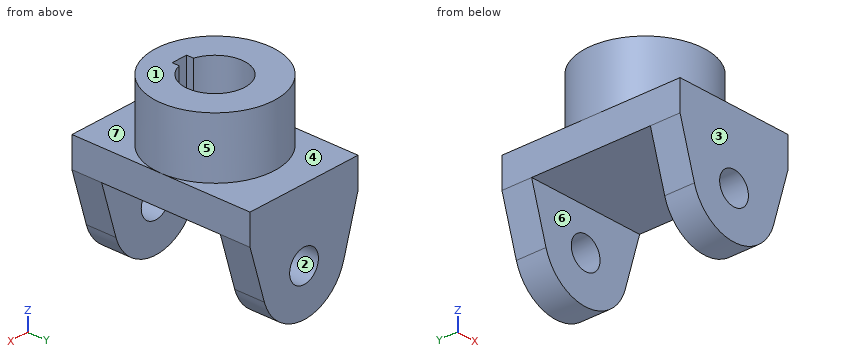
```python
from build123d import *

# Parameters (mm, degrees)
SKETCH1_W           = 60
SKETCH1_H           = 90
BOSS_EXTRUDE1_DEPTH = 7.5
SKETCH2_R           = 30
BOSS_EXTRUDE4_DEPTH = 30
SKETCH3_R           = 8
BOSS_EXTRUDE5_DEPTH = 15


with BuildPart() as part:
    # Sketch1 → Boss-Extrude1 (new body, symmetric)
    with BuildSketch(Plane.XY):
        Rectangle(SKETCH1_W, SKETCH1_H)
    extrude(amount=BOSS_EXTRUDE1_DEPTH, both=True)

    # Sketch2 → Boss-Extrude4 (add)
    with BuildSketch(Plane.XY.offset(7.5)):
        Circle(SKETCH2_R)
        with BuildLine():
            Line((4, -18), (0, -18))
            Line((0, -18), (-4, -18))
            Line((-4, -18), (-4, -15))
            Line((-4, -15), (-4, -14.456832295))
            ThreePointArc((-4, -14.456832295), (-9.082951062, 11.937336386), (15, 0))
            ThreePointArc((15, 0), (11.937336386, -9.082951062), (4, -14.456832295))
            Line((4, -14.456832295), (4, -18))
        make_face(mode=Mode.SUBTRACT)
    extrude(amount=BOSS_EXTRUDE4_DEPTH)

    # Sketch3 → Boss-Extrude5 (add)
    with BuildSketch(Plane(origin=(0, 45, 0), x_dir=(1, 0, 0), z_dir=(0, 1, 0))):
        with BuildLine():
            Line((-22.03289839, 34.099347585), (-30, 7.5))
            Line((-30, 7.5), (-11.357816691, 7.5))
            ThreePointArc((-11.357816691, 7.5), (-21.345170095, 18.933570545), (-22.03289839, 34.099347585))
        make_face()
        with BuildLine():
            Line((30, 7.5), (22.03289839, 34.099347585))
            ThreePointArc((22.03289839, 34.099347585), (22.756940293, 30.834916568), (23, 27.5))
            ThreePointArc((23, 27.5), (19.877497125, 15.929126738), (11.357816692, 7.5))
            Line((11.357816692, 7.5), (30, 7.5))
        make_face()
        with BuildLine():
            ThreePointArc((22.03289839, 34.099347585), (0, 50.5), (-22.03289839, 34.099347585))
            ThreePointArc((-22.03289839, 34.099347585), (-21.345170095, 18.933570545), (-11.357816691, 7.5))
            Line((-11.357816691, 7.5), (11.357816692, 7.5))
            ThreePointArc((11.357816692, 7.5), (19.877497125, 15.929126738), (23, 27.5))
            ThreePointArc((23, 27.5), (22.756940293, 30.834916568), (22.03289839, 34.099347585))
        make_face()
        with Locations((0, 27.5)):
            Circle(SKETCH3_R, mode=Mode.SUBTRACT)
    boss_extrude5 = extrude(amount=-BOSS_EXTRUDE5_DEPTH)

    # Mirror1: Boss-Extrude5 across plane
    add(boss_extrude5.mirror(Plane.ZX))


solid = part.part
```
Input: part model. Units: mm. Frame: model coordinates. Face numbers are marked on the shaded views. A direction names the side the tool comes from. Coordinates: 2 decimals unless noted, no trailing zeros. Loops run counter-clockwise (first coordinate to the right, second up) from the corner with the lowest first, then second, coordinate; pieces in that order, holes last. Notation, with made-up numbers: M 76,5 L 135,5 A12 ccw 135,16 Z; hole C -10,33.25 d3. An arc over 180 degrees is marked long. Answer in a Markdown table with one row per item.
1. Reachability of the marked faces 4, 5, 6 and 7 from +Z, -Z, +X, -X, +Y, -Y: full face, straight path, thin tool, end or side. Return the list, or none.
Response:
| item | result |
|---|---|
| face 4 | +Z, +Y |
| face 5 | +Z |
| face 6 | -Z, +X, -X |
| face 7 | +Z, -Y |
2. First-contact query: pin 1 (2 mm diameter, centred on x = 18.5, z = 14.5, fed in from +Y); pin 2 (2 mm diameter, centred on x = -12, z = 19.5, fed in from +Y); pin 3 (5 mm diameter, centred on x = -22.5, y = 14, fed in from -Z). Flat tips, straight axial feed; report the tip coordinate or a pass-through.
Response:
| item | result |
|---|---|
| pin 1 | stops at y = 24.37 |
| pin 2 | stops at y = 27.91 |
| pin 3 | stops at z = -7.5 |
3. Section C-C, the plane y = 18. Output: boundary loops of the cut face in (x, z), then the cut area to 3 significant figures.
Response:
| item | result |
|---|---|
| outline | M -30,-7.5 L 30,-7.5 L 30,7.5 L 24,7.5 L 24,37.5 L -24,37.5 L -24,7.5 L -30,7.5 Z |
| area | 2,340 mm2 |
4. Section D-D, the plane z = -27.5. Output: boundary loops of the cut face in (x, y), then the cut area to 3 significant figures.
Response:
| item | result |
|---|---|
| outline | M -24.01,-45 L -8,-45 L -8,-30 L -24.01,-30 Z; M -24.01,30 L -8,30 L -8,45 L -24.01,45 Z; M 8,-45 L 24.01,-45 L 24.01,-30 L 8,-30 Z; M 8,30 L 24.01,30 L 24.01,45 L 8,45 Z |
| area | 961 mm2 |
5. Draft query along Z for the marked faces 1, 2 and 3. Return one class per face: pulls with the +Z half, pulls with the -Z half, needs draft (parallel to the pull), parting line crosses it, or undercut.
Response:
| item | result |
|---|---|
| face 1 | pulls with the +Z half |
| face 2 | undercut |
| face 3 | needs draft |
6. Section B-B, the plane z = 31.5. Output: boundary loops of the cut face in (x, y).
Response:
| item | result |
|---|---|
| outline | C 0,0 d60; hole M -4,-18 L 4,-18 L 4,-14.46 A15 ccw long -4,-14.46 Z |
7. Material intervals for line 1 (Y direction, x = 0, z = 26); line 2 (Y direction, x = -6.5, z = -36.5); line 3 (Z direction, x = -0.5, y = 36), sorted ascending.
Response:
| item | result |
|---|---|
| line 1 | y = -30 to -18, 15 to 30 |
| line 2 | y = -45 to -30, 30 to 45 |
| line 3 | z = -50.49 to -35.48, -19.52 to 7.5 |
8. Section A-A, the plane x = 0. Output: boundary loops of the cut face in (y, z).
Response:
| item | result |
|---|---|
| outline | M -45,-50.5 L -30,-50.5 L -30,-35.5 L -45,-35.5 Z; M -45,-19.5 L -30,-19.5 L -30,-7.5 L 30,-7.5 L 30,-19.5 L 45,-19.5 L 45,7.5 L 30,7.5 L 30,37.5 L 15,37.5 L 15,7.5 L -18,7.5 L -18,37.5 L -30,37.5 L -30,7.5 L -45,7.5 Z; M 30,-50.5 L 45,-50.5 L 45,-35.5 L 30,-35.5 Z |
